from build123d import *

# Parameters (mm, degrees)
F2_DEPTH = 25.4
F3_DEPTH = 25.4
F4_DEPTH = 38.101
F0_W     = 16.933333
F0_H     = 6.35
F5_DEPTH = 25.4


with BuildPart() as f2:
    # F1 (on Right) → F2 (new body)
    with BuildSketch(Plane.YZ):
        Polygon((-38.1, 0), (0, 0), (0, 6.35), (-12.7, 6.35), (-25.4, 6.35), (-38.1, 6.35), align=None)
    extrude(amount=F2_DEPTH)

    # F1 (on Right) → F3 (join)
    with BuildSketch(Plane.YZ):
        Polygon((-12.7, 6.35), (0, 6.35), (0, 25.4), (-12.7, 25.4), (-12.7, 19.05), (-25.4, 19.05), (-25.4, 12.7), (-12.7, 12.7), align=None)
    extrude(amount=F3_DEPTH)

    # F0 (on Front) → F4 (cut, through all)
    with BuildSketch(Plane.XZ):
        Polygon((16.933333, 12.7), (25.4, 6.35), (25.4, 25.4), (0, 25.4), (8.466667, 19.05), align=None)
    extrude(amount=F4_DEPTH, mode=Mode.SUBTRACT)

    # F0 (on Front) → F5 (join)
    with BuildSketch(Plane.XZ):
        with Locations((8.466666, 9.525)):
            Rectangle(F0_W, F0_H)
    extrude(amount=F5_DEPTH)


solid = f2.part
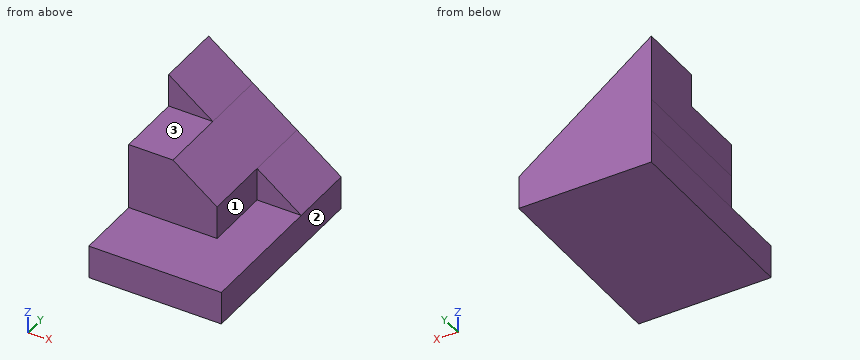
Can you work these out from the model? Positions are in its coordinate system, mm. Face numbers are marked on the shaded views. A direction names the side the tool comes from. Give positions to 0.01 mm unless a question says otherwise; leave off trailing zeros. Order: outer loops, then holes, each group sorted by start corner. A loop starts at its lowest first (then second) coordinate and runs counter-clockwise, first axis right, second up. Notation, with made-up numbers: M 2,55 L 60,55 A31 ccw 60,79 Z; hole C 12.25,9.25 d9. An arc over 180 degrees is marked long. Use one line per item in the form item = value.
Item 1: If we section it at B-B, the plane z = 7.25: Write out the boundary of the cut face in (x, y).
Values follow:
outline = M 0,-25.4 L 16.93,-25.4 L 16.93,-12.7 L 24.2,-12.7 L 24.2,0 L 0,0 Z
Item 2: If I drill on line 1 along Y through (x, z) = (2.25, 15); line 2 along Z through (x, y) = (23.5, -25.5); line 3 along X through (y, z) = (-21.5, 8.5), over which ranges is the centre line in solid material (lowest first)? Write a range as [from, to].
Values follow:
line_1 = [-25.4, 0]
line_2 = [0, 6.35]
line_3 = [0, 16.93]
Item 3: If we section it at C-C, the plane x = 7: Write out the boundary of the cut face in (y, z).
Values follow:
outline = M -38.1,0 L 0,0 L 0,20.15 L -12.7,20.15 L -12.7,19.05 L -25.4,19.05 L -25.4,6.35 L -38.1,6.35 Z
Item 4: If we section it at D-D, the plane y = -6: Write out the boundary of the cut face in (x, z).
Values follow:
outline = M 0,0 L 25.4,0 L 25.4,6.35 L 0,25.4 Z
Item 5: If we section it at A-A, the plane y = -19: Write out the boundary of the cut face in (x, z).
Values follow:
outline = M 0,0 L 25.4,0 L 25.4,6.35 L 16.93,6.35 L 16.93,12.7 L 8.47,19.05 L 0,19.05 Z
Item 6: Will these pins go through, and if not, where does the flat tip stop? pin 1 Ø14 at (x, z) = (8, 12) entering from -Y; pin 2 Ø10 at (x, y) = (12.5, -34) entering from +Z; pin 3 Ø8 at (x, z) = (4.5, 15.5) entering from -Y; pin 4 Ø6 at (y, z) = (-27.5, 20) entering from +X.
Values follow:
pin_1 = -38.1
pin_2 = 6.35
pin_3 = -25.4
pin_4 = 10.06
Item 7: For the marked faces 1, 2 and 3, which set-ups out of +Z, -Z, +X, -X, +Y, -Y let a thin tool reach every point of the face, with its end or its side?
Values follow:
face_1 = +Z, +X, -Y
face_2 = +Z, -Z, +X, +Y, -Y
face_3 = +Z, +X, -X, -Y
